```python
from build123d import *

# Parameters (mm, degrees)
SKETCH1_W           = 25.4
SKETCH1_H           = 203.2
BOSS_EXTRUDE1_DEPTH = 2.54
CUT_EXTRUDE1_DEPTH  = 1.27


with BuildPart() as part:
    # Sketch1 → Boss-Extrude1 (new body)
    with BuildSketch(Plane(origin=(0, 0, 0), x_dir=(1, 0, 0), z_dir=(0, 1, 0))):
        Rectangle(SKETCH1_W, SKETCH1_H)
    extrude(amount=-BOSS_EXTRUDE1_DEPTH)

    # Sketch3 → Cut-Extrude1 (cut)
    with BuildSketch(Plane(origin=(0, 0, 0), x_dir=(1, 0, 0), z_dir=(0, 1, 0))):
        Polygon((12.7, 40.64), (6.35, 34.29), (6.35, 67.31), (12.7, 60.96), align=None)
        Polygon((-6.35, 67.31), (-12.7, 60.96), (-12.7, 40.64), (-6.35, 34.29), align=None)
        Polygon((6.35, -67.31), (12.7, -60.96), (12.7, -40.64), (6.35, -34.29), align=None)
        Polygon((-6.35, -34.29), (-6.35, -67.31), (-12.7, -60.96), (-12.7, -40.64), align=None)
    extrude(amount=-CUT_EXTRUDE1_DEPTH, mode=Mode.SUBTRACT)


solid = part.part
```
The listing builds one solid part. Answer for the finished solid, in the listing's coordinates (mm). A direction names the side the tool comes from. Give positions to 0.01 mm unless a question says otherwise; leave off trailing zeros. Order: outer loops, then holes, each group sorted by start corner. A loop starts at its lowest first (then second) coordinate and runs counter-clockwise, first axis right, second up. Notation, with made-up numbers: (45.5, 21.25) - (84.5, 21.25) arc R14 ccw to (84.5, 36.25) - close; hole circle Ø6 at (49.5, 54.25). An arc over 180 degrees is marked (long way). Answer in a Markdown table with one row per item. Add a question column.
Q1. The part is cut by section A-A (z = 37). Determine the outline of the cut face in (x, y), then the cut area to 3 significant figures.
Q2. Find the intervals of material crossed by line 1 along Z through (x, y) = (-7, -0.75); line 2 along Z through (x, y) = (9.25, -0.25); line 3 along X through (y, z) = (-0.45, 50), in increasing order. Write a range as [from, to].
Q3. The part is cut by section C-C (y = -0.4). Determine the outline of the cut face in (x, z), then the cut area to 3 significant figures.
Q4. The part is cut by section B-B (x = 8). Determine the outline of the cut face in (y, z).
Q5. Given P1, Ø3, axis at x = -10.5, z = -45.5, coming from the +Y side, flat-ended and moving along its own axis, determine where the tip first touches the part or whether it passes through.
Q6. Which of the six approach directions +Z, -Z, +X, -X, +Y, -Y give full straight-line access (tool end or side, diameter ignored) to faces 1 (the flat face through (-10, -1.27, -51)), 2 (the flat face through (0, -2.54, -1))?
Determined:
| question | item | result |
|---|---|---|
| 1 | outline | (-12.7, -2.54) - (12.7, -2.54) - (12.7, 0) - (9.06, 0) - (9.06, -1.27) - (6.35, -1.27) - (6.35, 0) - (-6.35, 0) - (-6.35, -1.27) - (-9.06, -1.27) - (-9.06, 0) - (-12.7, 0) - close |
| 1 | area | 57.6 mm² |
| 2 | line 1 | z = [-101.6, -66.66], [-34.94, 34.94], [66.66, 101.6] |
| 2 | line 2 | z = [-101.6, -64.41], [-37.19, 37.19], [64.41, 101.6] |
| 2 | line 3 | x = [-6.35, 6.35] |
| 3 | outline | (-12.7, -101.6) - (12.7, -101.6) - (12.7, -60.96) - (6.35, -67.31) - (6.35, -34.29) - (12.7, -40.64) - (12.7, 40.64) - (6.35, 34.29) - (6.35, 67.31) - (12.7, 60.96) - (12.7, 101.6) - (-12.7, 101.6) - (-12.7, 60.96) - (-6.35, 67.31) - (-6.35, 34.29) - (-12.7, 40.64) - (-12.7, -40.64) - (-6.35, -34.29) - (-6.35, -67.31) - (-12.7, -60.96) - close |
| 3 | area | 4,480 mm² |
| 4 | outline | (-2.54, -101.6) - (0, -101.6) - (0, -65.66) - (-1.27, -65.66) - (-1.27, -35.94) - (0, -35.94) - (0, 35.94) - (-1.27, 35.94) - (-1.27, 65.66) - (0, 65.66) - (0, 101.6) - (-2.54, 101.6) - close |
| 5 | P1 | stops at y = -1.27 |
| 6 | face 1 | +Y |
| 6 | face 2 | +Z, -Z, +X, -X, -Y |
